Geometry check sheet. Reference: the model listing, model coordinates, mm. Give positions to 0.01 mm unless a question says otherwise; leave off trailing zeros. Order: outer loops, then holes, each group sorted by start corner. A loop starts at its lowest first (then second) coordinate and runs counter-clockwise, first axis right, second up. Notation, with made-up numbers: (66, 49) - (106, 49) arc R18 ccw to (106, 62) - close; hole circle Ø2 at (36, 2). An arc over 180 degrees is marked (long way). Put each result on its own line as item: value. Start each with the question number.
```python
from build123d import *

# Parameters (mm, degrees)
F1_DEPTH = 1.32
F2_D     = 2.75


with BuildPart() as f1:
    # F0 (on Top) → F1 (new body)
    with BuildSketch(Plane.XY):
        with BuildLine():
            ThreePointArc((42.5, 25), (41.62132, 27.12132), (39.5, 28))
            Line((39.5, 28), (-39.5, 28))
            ThreePointArc((-39.5, 28), (-41.62132, 27.12132), (-42.5, 25))
            Line((-42.5, 25), (-42.5, -25))
            ThreePointArc((-42.5, -25), (-41.62132, -27.12132), (-39.5, -28))
            Line((-39.5, -28), (39.5, -28))
            ThreePointArc((39.5, -28), (41.62132, -27.12132), (42.5, -25))
            Line((42.5, -25), (42.5, 25))
        make_face()
    extrude(amount=F1_DEPTH)

    # F2 (through all)
    with Locations(Plane(origin=(0, 0, 0), x_dir=(1, 0, 0), z_dir=(0, 0, -1))):
        with Locations((-39, 24.5), (10, 24.5), (10, -24.5), (-39, -24.5)):
            Hole(F2_D / 2)


solid = f1.part
```
Item 1: Cross-section at A-A (x = 10). Enter the section's corners in (y, z) (3 decimals), and give its area (3 significant figures).
Item 2: Release check for a two-part mould opening along Y. For faces 1 (the face through (-41.64, -27.1, 0.65)), 2 (the face through (41.64, 27.1, 0.65)), 3 (the face through (10.179, -25.863, 0.669)), 4 (the face through (-1, 0, 0)) record: +Y half, -Y half, draft (parallel to the pull), parting line (faces both ways), or undercut.
Item 3: Thickness scan on line 1 along X through (y, z) = (24.5, 0.3) (3 decimals); line 2 along Y through (x, z) = (-39, 0.8) (3 decimals); line 3 along X through (y, z) = (26, 0.65). Record the ranges inside material, lowest first.
Item 4: Gauge pin test, flat end, axial feed: pin 1 Ø1.6 at (x, y) = (10, -24.5) entering from +Z. Record the tip position at first contact, or that the pin passes through.
Recorded:
1. outline: (-28, 0) - (-25.875, 0) - (-25.875, 1.32) - (-28, 1.32) - close; (-23.125, 0) - (23.125, 0) - (23.125, 1.32) - (-23.125, 1.32) - close; (25.875, 0) - (28, 0) - (28, 1.32) - (25.875, 1.32) - close
1. area: 66.7 mm^2
2. face 1: -Y half
2. face 2: +Y half
2. face 3: undercut
2. face 4: draft
3. line 1: x = -42.5 to -40.375, -37.625 to 8.625, 11.375 to 42.5
3. line 2: y = -28 to -25.875, -23.125 to 23.125, 25.875 to 28
3. line 3: x = -42.33 to 42.33
4. pin 1: passes through
